from build123d import *

# Parameters (mm, degrees)
ESBO_O1_R                = 1.598160281
ESBO_O1_R_2              = 1.600993429
RESSALTO_EXTRUS_O1_DEPTH = 5
ESBO_O2_W                = 8.00000038
ESBO_O2_H                = 10.097505558
RESSALTO_EXTRUS_O2_DEPTH = 17.65
ESBO_O3_W                = 7
ESBO_O3_H                = 10.097505558
RESSALTO_EXTRUS_O3_DEPTH = 15.515714
ESBO_O4_R                = 3
CORTE_EXTRUS_O1_DEPTH    = 13
ESBO_O5_W                = 7.0157148
ESBO_O5_H                = 10.097505558
RESSALTO_EXTRUS_O4_DEPTH = 30
ESBO_O6_R                = 3
CORTE_EXTRUS_O2_DEPTH    = 30


with BuildPart() as part:
    # Esboço1 → Ressalto-extrusão1 (new body)
    with BuildSketch(Plane.XY):
        with BuildLine():
            Line((-10.199065979, -3.817665654), (-4.00000019, -5.764999893))
            Line((-4.00000019, -5.764999893), (4.00000019, -5.764999893))
            Line((4.00000019, -5.764999893), (10.197782, -3.817301838))
            ThreePointArc((10.197782, -3.817301838), (12.999977706, 0.001566069), (10.195969576, 3.8191034))
            Line((10.195969576, 3.8191034), (4.00000019, 5.763000809))
            Line((4.00000019, 5.763000809), (-4.00000019, 5.763000809))
            Line((-4.00000019, 5.763000809), (-10.199143851, 3.815503142))
            ThreePointArc((-10.199143851, 3.815503142), (-13.000622723, -0.001109837), (-10.199065979, -3.817665654))
        make_face()
        with Locations((8.997973452, 0.000616233)):
            Circle(ESBO_O1_R, mode=Mode.SUBTRACT)
        with Locations((-9.000145119, -0.001069025)):
            Circle(ESBO_O1_R_2, mode=Mode.SUBTRACT)
    extrude(amount=RESSALTO_EXTRUS_O1_DEPTH)

    # Esboço2 → Ressalto-extrusão2 (add)
    with BuildSketch(Plane.XY.offset(5)):
        with Locations((0, 0.71424803)):
            Rectangle(ESBO_O2_W, ESBO_O2_H)
    extrude(amount=RESSALTO_EXTRUS_O2_DEPTH)

    # Esboço3 → Ressalto-extrusão3 (add)
    with BuildSketch(Plane.ZY.offset(4.00000019)):
        with Locations((19.15, 0.71424803)):
            Rectangle(ESBO_O3_W, ESBO_O3_H)
    extrude(amount=RESSALTO_EXTRUS_O3_DEPTH)

    # Esboço4 → Corte-extrusão1 (cut)
    with BuildSketch(Plane(origin=(0, 0, 15.65), x_dir=(-1, 0, 0), z_dir=(0, 0, -1))):
        with Locations((15.448687317, 0.71424803)):
            Circle(ESBO_O4_R)
    extrude(amount=-CORTE_EXTRUS_O1_DEPTH, mode=Mode.SUBTRACT)

    # Esboço5 → Ressalto-extrusão4 (add)
    with BuildSketch(Plane.XY.offset(22.65)):
        with Locations((0.49214279, 0.71424803)):
            Rectangle(ESBO_O5_W, ESBO_O5_H)
    extrude(amount=RESSALTO_EXTRUS_O4_DEPTH)

    # Esboço6 → Corte-extrusão2 (cut)
    with BuildSketch(Plane(origin=(4.00000019, 0, 0), x_dir=(0, 0, -1), z_dir=(1, 0, 0))):
        with Locations((-48.08055434, 0.71424803)):
            Circle(ESBO_O6_R)
    extrude(amount=-CORTE_EXTRUS_O2_DEPTH, mode=Mode.SUBTRACT)


solid = part.part
Source: CAD feature listing. Evaluate the final solid. Frame: model axes, mm. A direction names the side the tool comes from. Coordinates: 2 decimals unless noted, no trailing zeros. Order: outer loops, then holes, each group sorted by start corner. A loop starts at its lowest first (then second) coordinate and runs counter-clockwise, first axis right, second up. Notation, with made-up numbers: M -5.5,-2 L 44.5,-2 A7 ccw 44.5,3 Z; hole C 50.25,71 d7. An arc over 180 degrees is marked long. Write each question's results on one line, items separated by ' | '. Start each with the question number.
1. Section B-B, the plane y = 2.5. Return the cut outline in (x, z).
2. Section D-D, the plane x = -5. Return the cut outline in (y, z).
3. Material intervals for L1, parallel to X at y = 0.25, z = 4; L2, parallel to Z at x = -12, y = -0.5; L3, parallel to Y at x = -1, z = 48, sorted ascending.
4. Pin query (flat end, axial travel): pin 1 (2 mm diameter, centred on x = 2.5, y = -0.5, fed in from -Z); pin 2 (5.5 mm diameter, centred on y = 0.71, z = 48.08, fed in from +X); pin 3 (5 mm diameter, centred on x = -9, y = 0.5, fed in from +Z); pin 4 (5 mm diameter, centred on y = 0, z = 38, fed in from -X). Return the tip coordinate at first contact, or that it passes through.
5. Section A-A, the plane x = -9. Return the cut outline in (y, z), then the cut area to 3 significant figures.
6. Draft query along Z for faces 1 (the face through (-13, 0, 2)), 2 (the face through (0, -5, 5)), 3 (the face through (-11, 1, 22.65)). Return one class per face: +Z half, -Z half, draft (parallel to the pull), parting line (faces both ways), or undercut.
7. Reachability of faces 4 (the face through (-7.473, 0.48, 2.465)), 5 (the face through (4, 1, 28)), 6 (the face through (-7.14, -4.78, 2.46)), 7 (the face through (-4, 1, 10)), 8 (the face through (-3.016, 1, 37)) from +Z, -Z, +X, -X, +Y, -Y: full face, straight path, thin tool, end or side. Return the list, or none.
Solution:
1) outline: M -19.52,15.65 L -17.86,15.65 L -17.86,22.65 L -19.52,22.65 Z; M -13.04,15.65 L -4,15.65 L -4,5 L -12.12,5 L -12.12,0 L 12.12,0 L 12.12,5 L 4,5 L 4,45.67 L -3.02,45.67 L -3.02,22.65 L -13.04,22.65 Z; M -3.02,50.49 L 4,50.49 L 4,52.65 L -3.02,52.65 Z
2) outline: M -5.45,0 L 5.45,0 L 5.45,5 L -5.45,5 Z; M -4.33,15.65 L 5.76,15.65 L 5.76,22.65 L -4.33,22.65 Z
3) L1: -12.99 to -10.58, -7.42 to 7.42, 10.58 to 12.99 | L2: 0 to 5, 15.65 to 22.65 | L3: -4.33 to -2.28, 3.71 to 5.76
4) pin 1: z = 0 | pin 2: through | pin 3: z = 22.65 | pin 4: x = -3.02
5) outline: M -4.33,15.65 L 5.76,15.65 L 5.76,22.65 L -4.33,22.65 Z; M -4.19,0 L -1.6,0 L -1.6,5 L -4.19,5 Z; M 1.6,0 L 4.19,0 L 4.19,5 L 1.6,5 Z | area: 96.6 mm²
6) face 1: draft | face 2: undercut | face 3: +Z half
7) face 4: -Z | face 5: +Z, +X, +Y, -Y | face 6: -Z, -X, -Y | face 7: -X, +Y, -Y | face 8: +Z, -X, +Y, -Y
